Model file for the job. Use its own axes, mm. Coordinates: 2 decimals unless noted, no trailing zeros. Order: outer loops, then holes, each group sorted by start corner. A loop starts at its lowest first (then second) coordinate and runs counter-clockwise, first axis right, second up. Notation, with made-up numbers: (72, 11) -> (94, 11) arc R21 cw to (94, 49) -> close; hole circle Ø11 at (14, 64). An arc over 180 degrees is marked (long way). Use CSV: the item, a comma, the result in double quotes. Start each with the question number.
(1) Cut at C-C on z = -3.75. Write the cut outline in (x, y).
(2) Probe L1, parallel to X at y = 0.4, z = -3.5; L2, parallel to X at y = 0.15, z = -3.75; L3, parallel to Z at x = 3, y = 0.25. List the from-to ranges inside material, lowest first.
(3) Cut at B-B on x = -2.75. Write the cut outline in (y, z), plus the area to 3 significant figures.
(4) Cut at A-A on y = 0.15. Write the cut outline in (x, z), plus the area to 3 significant figures.
Autodesk Inventor part; units mm, degrees
ref_plane "YZ Plane" through (0, 0, 0) normal (1, 0, 0) x (0, 1, 0)
ref_plane "XZ Plane" through (0, 0, 0) normal (0, 1, 0) x (-1, 0, 0)
ref_plane "XY Plane" through (0, 0, 0) normal (0, 0, 1) x (1, 0, 0)
sketch "Sketch1" plane through (0, 0, 0) normal (0, 1, 0) x (-1, 0, 0)
  line L0 (0, -5.2573) -> (-3.0902, -4.2533) construction
  line L1 (-3.0902, -4.2533) -> (-5, -1.6246) construction
  line L2 (-5, -1.6246) -> (-5, 1.6246) construction
  line L3 (-5, 1.6246) -> (-3.0902, 4.2533) construction
  line L4 (-3.0902, 4.2533) -> (0, 5.2573) construction
  line L5 (0, 5.2573) -> (3.0902, 4.2533) construction
  line L6 (3.0902, 4.2533) -> (5, 1.6246) construction
  line L7 (5, 1.6246) -> (5, -1.6246) construction
  line L8 (5, -1.6246) -> (3.0902, -4.2533) construction
  line L9 (3.0902, -4.2533) -> (0, -5.2573) construction
  line L10 (-2.0711, -5) -> (-5, -2.0711)
  line L11 (-5, -2.0711) -> (-5, 2.0711)
  line L12 (-5, 2.0711) -> (-2.0711, 5)
  line L13 (-2.0711, 5) -> (2.0711, 5)
  line L14 (2.0711, 5) -> (5, 2.0711)
  line L15 (5, 2.0711) -> (5, -2.0711)
  line L16 (5, -2.0711) -> (2.0711, -5)
  line L17 (2.0711, -5) -> (-2.0711, -5)
  line L18 (0, 0) -> (-10.1721, 0) construction
  dimension "d0" = 10
  dimension "d3" = 10
extrude "Extrusion1" add sketch "Sketch1" along normal blind 0.5
properties part number "Substrate"
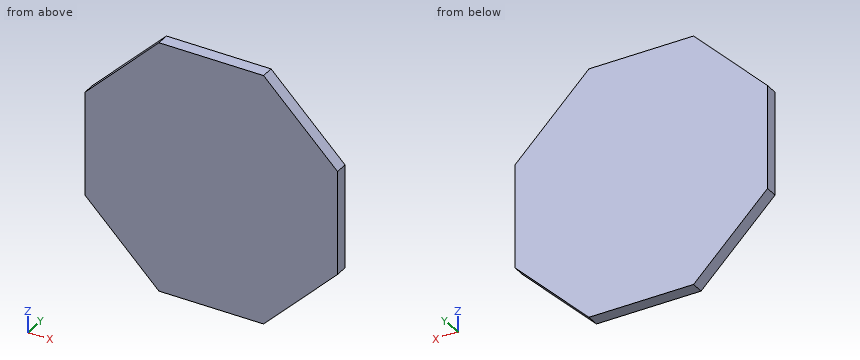
Outcome:
1,outline,"(-3.32, 0) -> (3.32, 0) -> (3.32, 0.5) -> (-3.32, 0.5) -> close"
2,L1,"-3.57 to 3.57"
2,L2,"-3.32 to 3.32"
2,L3,"-4.07 to 4.07"
3,outline,"(0, -4.32) -> (0.5, -4.32) -> (0.5, 4.32) -> (0, 4.32) -> close"
3,area,"4.32 mm2"
4,outline,"(-5, -2.07) -> (-2.07, -5) -> (2.07, -5) -> (5, -2.07) -> (5, 2.07) -> (2.07, 5) -> (-2.07, 5) -> (-5, 2.07) -> close"
4,area,"82.8 mm2"
